```python
from build123d import *

# Parameters (mm, degrees)
SKETCH1_W                   = 25.4
SKETCH1_H                   = 63.5
BOSS_EXTRUDE1_DEPTH         = 111.37596
F_1_4_0_25_DIAMETER_HOLE1_D = 6.35
F_6_0MM_DOWEL_HOLE1_D       = 6.3
F_6_0MM_DOWEL_HOLE1_DEPTH   = 9.0000074
F_6_0MM_DOWEL_HOLE1_TIP     = 1.89271095


with BuildPart() as part:
    # Sketch1 → Boss-Extrude1 (new body)
    with BuildSketch(Plane(origin=(0, 0, 0), x_dir=(0, 0, -1), z_dir=(1, 0, 0))):
        with Locations((12.7, 31.75)):
            Rectangle(SKETCH1_W, SKETCH1_H)
    extrude(amount=-BOSS_EXTRUDE1_DEPTH)

    # 1/4 (0.25) Diameter Hole1 (through all)
    with Locations(Plane.XY):
        with Locations((-98.67596, 32), (-47.87596, 32), (-73.27596, 32)):
            Hole(F_1_4_0_25_DIAMETER_HOLE1_D / 2)

    # Ø6.0mm Dowel Hole1
    with Locations(Plane(origin=(0, 0, 0), x_dir=(0, 0, -1), z_dir=(1, 0, 0))):
        with Locations((15.4, 7), (15.4, 53)):
            Hole(F_6_0MM_DOWEL_HOLE1_D / 2, depth=F_6_0MM_DOWEL_HOLE1_DEPTH)
            with Locations((0, 0, -(F_6_0MM_DOWEL_HOLE1_DEPTH + F_6_0MM_DOWEL_HOLE1_TIP / 2))):  # 118° drill point
                Cone(0, F_6_0MM_DOWEL_HOLE1_D / 2, F_6_0MM_DOWEL_HOLE1_TIP, mode=Mode.SUBTRACT)


solid = part.part
```
Geometry: final body of the model. Coordinates: model frame, mm. A direction names the side the tool comes from. Round coordinates to 2 decimals unless told otherwise and drop trailing zeros. Write each loop counter-clockwise with the first axis right and the second up, starting at its lowest first coordinate (ties: lowest second). Pieces come first, ordered by that corner, then holes. Notation, with made-up numbers: (37.25, -21.75) -> (65.25, -21.75) arc R15 cw to (65.25, -4.75) -> close; hole circle Ø11 at (-26.5, 51.5). An arc over 180 degrees is marked (long way). Return JSON: item names as keys, results as strings.
Q1. Mould query, pull axis X, two halves, no side actions, for faces 3 (the flat face through (-55, 31, -25.4)), 4 (the cylindrical face through (-74.741, 29.183, -12.878)), 5 (the flat face through (-111.376, 32, -13)). Classes: +X half, -X half, draft (parallel to the pull), parting line (faces both ways), or undercut.
From the geometry:
{"face 3": "draft", "face 4": "undercut", "face 5": "-X half"}
Q2. Section A-A on x = -100. Return the cut outline in (y, z).
From the geometry:
{"outline": "(0, -25.4) -> (29.11, -25.4) -> (29.11, 0) -> (0, 0) -> close; (34.89, -25.4) -> (63.5, -25.4) -> (63.5, 0) -> (34.89, 0) -> close"}
Q3. Section B-B on z = -13.5. Give the number of separate pieces and of enclosed holes in the cut face, and give its area (3 significant figures).
From the geometry:
{"separate pieces": "1", "enclosed holes": "3", "area": "6,880 mm2"}
Q4. First-contact query: pin 1 Ø6 at (x, y) = (-82.5, 35) entering from +Z; pin 2 Ø5 at (x, y) = (-73.28, 32) entering from +Z; pin 3 Ø5.5 at (y, z) = (7, -15.4) entering from +X. Flat tips, straight axial feed; report the tip coordinate or a pass-through.
From the geometry:
{"pin 1": "z = 0", "pin 2": "through", "pin 3": "x = -9.24"}
Q5. Ray query, line 1 (Y direction, x = -6, z = -15.4); line 2 (Z direction, x = -6, y = 7); line 3 (Y direction, x = -5, z = -18.25). Return the intervals inside material, ascending.
From the geometry:
{"line 1": "0 to 3.85, 10.15 to 49.85, 56.15 to 63.5", "line 2": "-25.4 to -18.55, -12.25 to 0", "line 3": "0 to 5.66, 8.34 to 51.66, 54.34 to 63.5"}
Q6. Set-up query: faces 1 (the cylindrical face through (-4.563, 50.205, -13.946)), 2 (the flat face through (-55, 63.5, -13)). Return all of +Z, -Z, +X, -X, +Y, -Y with unobstructed straight access to the full face (end or side cutting, diameter ignored); none if empty.
From the geometry:
{"face 1": "+X", "face 2": "+Z, -Z, +X, -X, +Y"}
